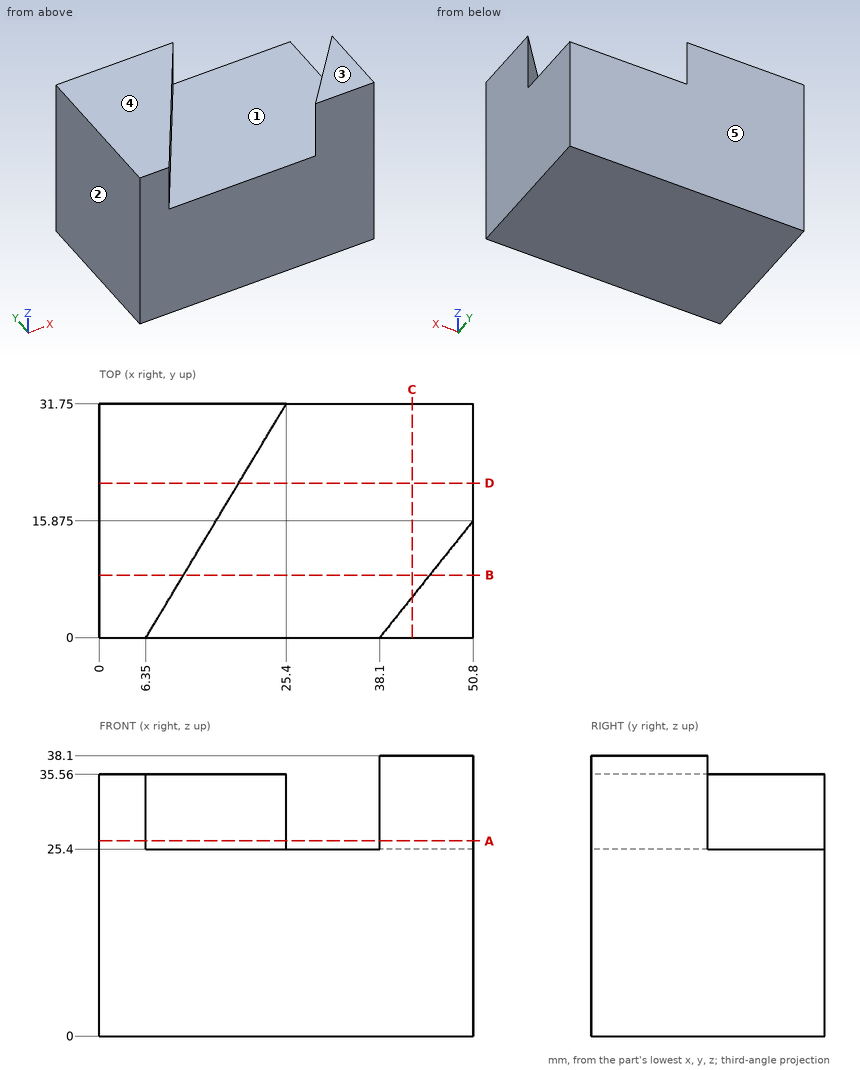
Here's the drawing with two shaded views (mm, measured from the low corner). I have some questions. A direction names the side the tool comes from. Give positions to 0.01 mm unless a question says otherwise; leave off trailing zeros. Loops run counter-clockwise (first coordinate to the right, second up) from the corner with the lowest first, then second, coordinate; pieces in that order, holes last. Notation, with made-up numbers: M -19,-19 L -10,-19 A21 cw -10,14 Z; hole C 50.25,34 d4. An arc over 180 degrees is marked long. One line per item, written item: value. Start each with the question number.
1) If we section it at D-D, the plane y = 21: Write out the boundary of the cut face in (x, z).
2) I'm going to push flat-ended pins straight in: pin 1 (9.5 mm diameter, centred on x = 22, y = 15, fed in from +Z); pin 2 (4 mm diameter, centred on x = 45.5, z = 31.5, fed in from +Y); pin 3 (7.5 mm diameter, centred on x = 16.5, y = 20.5, fed in from +Z). Where does each tip first touch, or does it pass through?
3) On a 3-axis mill with a long thin cutter (end or side, diameter ignored), from which of +Z, -Z, +X, -X, +Y, -Y can I reach the whole of each face in a straight line? I mean the marked faces 4 and 5. Say none if no direction works.
4) Thinking about a two-plate mould opening in X: for the marked faces 1, 2 and 3, which applies, +X half, -X half, draft (parallel to the pull), parting line (faces both ways), or undercut?
5) If we section it at B-B, the plane y = 8.5: Write out the boundary of the cut face in (x, z).
6) If we section it at A-A, the plane z = 26.5: Write out the boundary of the cut face in (x, y) (3 decimals), and give its area (3 significant figures).
7) If we section it at C-C, the plane x = 42.5: Write out the boundary of the cut face in (y, z).
8) If I drill on line 1 (Z direction, x = 3, y = 8); line 2 (X direction, y = 15, z = 28); line 3 (Z direction, x = 39.5, y = 29), over which ranges is the centre line in solid material (lowest first)? Write a range as [from, to].
Completed:
1. outline: M 0,0 L 50.8,0 L 50.8,25.4 L 18.95,25.4 L 18.95,35.56 L 0,35.56 Z
2. pin 1: stops at z = 25.4
2. pin 2: stops at y = 11.75
2. pin 3: stops at z = 35.56
3. face 4: +Z, -X, +Y, -Y
3. face 5: +Z, -Z, +X, -X, +Y
4. face 1: undercut
4. face 2: -X half
4. face 3: draft
5. outline: M 0,0 L 50.8,0 L 50.8,38.1 L 44.9,38.1 L 44.9,25.4 L 11.45,25.4 L 11.45,35.56 L 0,35.56 Z
6. outline: M 0,0 L 6.35,0 L 25.4,31.75 L 0,31.75 Z; M 38.1,0 L 50.8,0 L 50.8,15.875 Z
6. area: 605 mm^2
7. outline: M 0,0 L 31.75,0 L 31.75,25.4 L 5.5,25.4 L 5.5,38.1 L 0,38.1 Z
8. line 1: z = [0, 35.56]
8. line 2: x = [0, 15.35], [50.1, 50.8]
8. line 3: z = [0, 25.4]
